```python
from build123d import *

# Parameters (mm, degrees)
ESTRUSIONE_ESTRUSIONE1_DEPTH = 5
SCHIZZO2_W                   = 7.6
SCHIZZO2_H                   = 7.6
ESTRUSIONE_ESTRUSIONE2_DEPTH = 0.8
SCHIZZO3_R                   = 0.25
TAGLIO_ESTRUSIONE1_DEPTH     = 13.127654349
SCHIZZO4_R                   = 10
ESTRUSIONE_ESTRUSIONE3_DEPTH = 2
SMUSSO1_SIZE                 = 0.5


with BuildPart() as part:
    # Schizzo1 → Estrusione-Estrusione1 (new body)
    with BuildSketch(Plane(origin=(0, 0, 0), x_dir=(1, 0, 0), z_dir=(0, 1, 0))):
        with BuildLine():
            Line((-3.31662479, 5), (3.31662479, 5))
            ThreePointArc((3.31662479, 5), (6, 0), (3.31662479, -5))
            Line((3.31662479, -5), (-3.31662479, -5))
            ThreePointArc((-3.31662479, -5), (-6, 0), (-3.31662479, 5))
        make_face()
    extrude(amount=ESTRUSIONE_ESTRUSIONE1_DEPTH)

    # Schizzo2 → Estrusione-Estrusione2 (add)
    with BuildSketch(Plane(origin=(0, 5, 0), x_dir=(1, 0, 0), z_dir=(0, 1, 0))):
        Rectangle(SCHIZZO2_W, SCHIZZO2_H)
    extrude(amount=ESTRUSIONE_ESTRUSIONE2_DEPTH)

    # Schizzo3 → Taglio-Estrusione1 (cut, through all)
    with BuildSketch(Plane.XY.offset(3.8)):
        with Locations((0, 5.5)):
            Circle(SCHIZZO3_R)
    extrude(amount=-TAGLIO_ESTRUSIONE1_DEPTH, mode=Mode.SUBTRACT)

    # Schizzo4 → Estrusione-Estrusione3 (add)
    with BuildSketch(Plane.XZ):
        with Locations(Location((0, 0, 0), (0, 0, 270))):
            Circle(SCHIZZO4_R)
    extrude(amount=ESTRUSIONE_ESTRUSIONE3_DEPTH)

    # Smusso1
    smusso1_edges = [part.edges().sort_by_distance(p)[0] for p in [
        (0, 0, 10),
    ]]
    chamfer(smusso1_edges, length=SMUSSO1_SIZE)


solid = part.part
```
Can you work these out from the model? Positions are in its coordinate system, mm. A direction names the side the tool comes from. Coordinates: 2 decimals unless noted, no trailing zeros. Write each loop counter-clockwise with the first axis right and the second up, starting at its lowest first coordinate (ties: lowest second). Pieces come first, ordered by that corner, then holes. Notation, with made-up numbers: (21, 77.25) - (47, 77.25) arc R29 cw to (47, 101.25) - close; hole circle Ø4 at (50.25, 5). An arc over 180 degrees is marked (long way). Return JSON: item names as keys, results as strings.
Q1. I'm going to push flat-ended pins straight in: pin 1 Ø3 at (y, z) = (3.5, -3.5) entering from +X; pin 2 Ø3 at (x, y) = (-3, -1) entering from -Z; pin 3 Ø0.6 at (y, z) = (5.5, -1) entering from +X. Where does each tip first touch, or does it pass through?
Computed values:
{"pin 1": "stops at x = 5.66", "pin 2": "stops at z = -9.89", "pin 3": "stops at x = 3.8"}
Q2. On a 3-axis mill with a long thin cutter (end or side, diameter ignored), from which of +Z, -Z, +X, -X, +Y, -Y can I reach the whole of each face in a straight line? I mean faces 1 (the cylindrical face through (-6, 2, 0)), 2 (the flat face through (0, 2, 5)), 3 (the flat face through (0, 2, -5)), 4 (the cylindrical face through (6, 2, 0)). Say none if no direction works.
Computed values:
{"face 1": "-X, +Y", "face 2": "+Z, +X, -X, +Y", "face 3": "-Z, +X, -X, +Y", "face 4": "+X, +Y"}
Q3. If we section it at C-C (y = 5.5): Please give me the cut outline in (x, z).
Computed values:
{"outline": "(-3.8, -3.8) - (-0.25, -3.8) - (-0.25, 3.8) - (-3.8, 3.8) - close; (0.25, -3.8) - (3.8, -3.8) - (3.8, 3.8) - (0.25, 3.8) - close"}
Q4. Please list where these lines run through material, in increasing order: L1, parallel to Y at x = -4.75, z = 3; L2, parallel to Z at x = -0.25, y = 2.5; L3, parallel to Y at x = -5, z = -6.25. Write a range as from..to.
Computed values:
{"L1": "y = -2..5", "L2": "z = -5..5", "L3": "y = -2..0"}
Q5. If we section it at B-B (x = 0): Please give me the cut outline in (y, z).
Computed values:
{"outline": "(-2, -10) - (-0.5, -10) - (0, -9.5) - (0, -5) - (5, -5) - (5, -3.8) - (5.25, -3.8) - (5.25, 3.8) - (5, 3.8) - (5, 5) - (0, 5) - (0, 9.5) - (-0.5, 10) - (-2, 10) - close; (5.75, -3.8) - (5.8, -3.8) - (5.8, 3.8) - (5.75, 3.8) - close"}
Q6. If we section it at A-A (z = 0): Please give me the cut outline in (x, y).
Computed values:
{"outline": "(-10, -2) - (10, -2) - (10, -0.5) - (9.5, 0) - (6, 0) - (6, 5) - (3.8, 5) - (3.8, 5.8) - (-3.8, 5.8) - (-3.8, 5) - (-6, 5) - (-6, 0) - (-9.5, 0) - (-10, -0.5) - close; hole circle Ø0.5 at (0, 5.5)"}
Q7. If we section it at D-D (y = -0.25): Please give me the cut outline in (x, z), then the cut area to 3 significant figures.
Computed values:
{"outline": "circle Ø19.5 at (0, 0)", "area": "299 mm2"}
